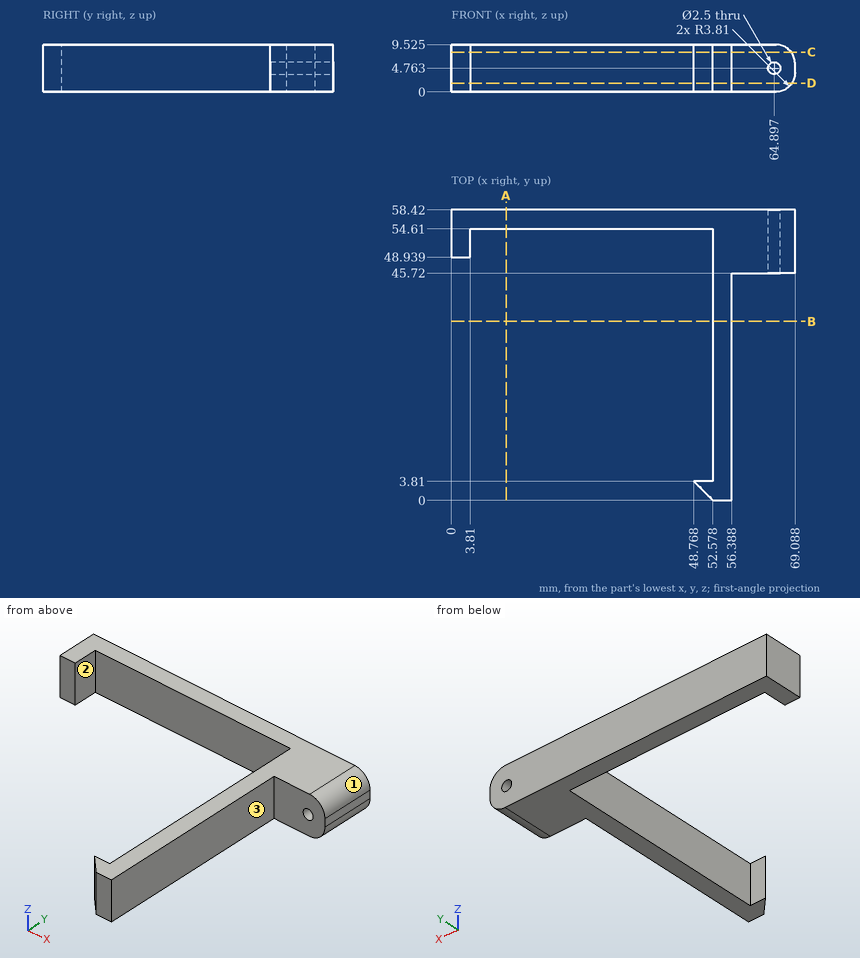
Geometry check sheet. Reference: drawing and pictorial views, mm from the part's lowest x, y, z. A direction names the side the tool comes from. Coordinates: 2 decimals unless noted, no trailing zeros. Order: outer loops, then holes, each group sorted by start corner. A loop starts at its lowest first (then second) coordinate and runs counter-clockwise, first axis right, second up.
Item 1: Depth check by flat-ended pin: pin 1 (2 mm diameter, centred on y = 42.5, z = 7, fed in from +X); pin 2 (2 mm diameter, centred on x = 64.9, z = 4.76, fed in from -Y); pin 3 (5 mm diameter, centred on x = 24.5, z = 6, fed in from -Y); pin 4 (1.9 mm diameter, centred on x = 2.5, z = 2.5, fed in from -Y). Enter the tip coordinate at first touch or a pass-through.
Filled in:
pin 1: stops at x = 56.39
pin 2: passes through
pin 3: stops at y = 54.61
pin 4: stops at y = 48.94
Item 2: Access from +Z, -Z, +X, -X, +Y, -Y to the whole of each face (thin tool, end or side, straight path). Record for the marked faces 1, 2 and 3.
Filled in:
face 1: +Z, +X, +Y, -Y
face 2: +Z, -Z, -Y
face 3: +Z, -Z, +X, -Y
Item 3: Material ranges on L1, parallel to X at y = 49, z = 4 (1 decimal); L2, parallel to Y at x = 61, z = 5.25; L3, parallel to X at y = 42.5, z = 0.5, recorded low to high.
Filled in:
L1: x = 0 to 3.8, 52.6 to 63.9, 65.9 to 69.1
L2: y = 45.72 to 58.42
L3: x = 52.58 to 56.39
Item 4: Section check C-C, the plane z = 8. Enter the section's corners in (x, y).
Filled in:
outline: (0, 48.94) - (3.81, 48.94) - (3.81, 54.61) - (52.58, 54.61) - (52.58, 3.81) - (48.77, 3.81) - (52.58, 0) - (56.39, 0) - (56.39, 45.72) - (68.33, 45.72) - (68.33, 58.42) - (0, 58.42) - close
Item 5: Section check B-B, the plane y = 36. Enter the section's corners in (x, z) (1 decimal).
Filled in:
outline: (52.6, 0) - (56.4, 0) - (56.4, 9.5) - (52.6, 9.5) - close
Item 6: Section check A-A, the plane x = 11. Enter the section's corners in (y, z) (1 decimal).
Filled in:
outline: (54.6, 0) - (58.4, 0) - (58.4, 9.5) - (54.6, 9.5) - close
Item 7: Section check D-D, the plane z = 1.75. Enter the section's corners in (x, y).
Filled in:
outline: (0, 48.94) - (3.81, 48.94) - (3.81, 54.61) - (52.58, 54.61) - (52.58, 3.81) - (48.77, 3.81) - (52.58, 0) - (56.39, 0) - (56.39, 45.72) - (68.48, 45.72) - (68.48, 58.42) - (0, 58.42) - close
